Source: CAD feature listing. Evaluate the final solid. Frame: model axes, mm. A direction names the side the tool comes from. Give positions to 0.01 mm unless a question says otherwise; leave off trailing zeros. Loops run counter-clockwise (first coordinate to the right, second up) from the corner with the lowest first, then second, coordinate; pieces in that order, holes last.
```python
from build123d import *

# Parameters (mm, degrees)
SKETCH1_R           = 1.45
SKETCH1_R_2         = 2.6
BOSS_EXTRUDE1_DEPTH = 3
SKETCH1_3_R         = 1.45
BOSS_EXTRUDE2_DEPTH = 29.5
SKETCH1_4_R         = 3
SKETCH1_4_R_2       = 1.45
BOSS_EXTRUDE3_DEPTH = 4
SKETCH5_W           = 14
SKETCH5_H           = 13
SKETCH5_W_2         = 16
SKETCH5_H_2         = 35
CUT_EXTRUDE2_DEPTH  = 3
CUT_EXTRUDE3_REACH  = 150.46


with BuildPart() as part:
    # Sketch1 → Boss-Extrude1 (new body)
    with BuildSketch(Plane.XY):
        with BuildLine():
            Line((-63.5, -59), (63.5, -59))
            ThreePointArc((63.5, -59), (65.621320344, -58.121320344), (66.5, -56))
            Line((66.5, -56), (66.5, 56))
            ThreePointArc((66.5, 56), (65.621320344, 58.121320344), (63.5, 59))
            Line((63.5, 59), (-63.5, 59))
            ThreePointArc((-63.5, 59), (-65.621320344, 58.121320344), (-66.5, 56))
            Line((-66.5, 56), (-66.5, -56))
            ThreePointArc((-66.5, -56), (-65.621320344, -58.121320344), (-63.5, -59))
        make_face()
        with Locations((-59.9, 40.875)):
            Circle(SKETCH1_R, mode=Mode.SUBTRACT)
        with Locations((33.1, 40.875)):
            Circle(SKETCH1_R, mode=Mode.SUBTRACT)
        with Locations((33.1, -30.875)):
            Circle(SKETCH1_R, mode=Mode.SUBTRACT)
        with Locations((-59.9, -30.875)):
            Circle(SKETCH1_R, mode=Mode.SUBTRACT)
        with Locations((-49.9, 11)):
            Circle(SKETCH1_R_2, mode=Mode.SUBTRACT)
        with Locations((51.5, 11)):
            Circle(SKETCH1_R_2, mode=Mode.SUBTRACT)
        with Locations((-49.9, -49)):
            Circle(SKETCH1_R_2, mode=Mode.SUBTRACT)
        with Locations((51.5, -49)):
            Circle(SKETCH1_R_2, mode=Mode.SUBTRACT)
        with BuildLine():
            Line((44.9, 26), (44.9, -16))
            ThreePointArc((44.9, -16), (43.435533906, -19.535533906), (39.9, -21))
            Line((39.9, -21), (9.9, -21))
            ThreePointArc((9.9, -21), (6.364466094, -19.535533906), (4.9, -16))
            Line((4.9, -16), (4.9, 26))
            ThreePointArc((4.9, 26), (6.364466094, 29.535533906), (9.9, 31))
            Line((9.9, 31), (39.9, 31))
            ThreePointArc((39.9, 31), (43.435533906, 29.535533906), (44.9, 26))
        make_face(mode=Mode.SUBTRACT)
        with BuildLine():
            Line((-39.9, 31), (-9.9, 31))
            ThreePointArc((-9.9, 31), (-6.364466094, 29.535533906), (-4.9, 26))
            Line((-4.9, 26), (-4.9, -16))
            ThreePointArc((-4.9, -16), (-6.364466094, -19.535533906), (-9.9, -21))
            Line((-9.9, -21), (-39.9, -21))
            ThreePointArc((-39.9, -21), (-43.435533906, -19.535533906), (-44.9, -16))
            Line((-44.9, -16), (-44.9, 26))
            ThreePointArc((-44.9, 26), (-43.435533906, 29.535533906), (-39.9, 31))
        make_face(mode=Mode.SUBTRACT)
    extrude(amount=-BOSS_EXTRUDE1_DEPTH)

    # Sketch1<3> → Boss-Extrude2 (add)
    with BuildSketch(Plane.XY):
        with BuildLine():
            ThreePointArc((-66.5, 56), (-65.621320344, 58.121320344), (-63.5, 59))
            Line((-63.5, 59), (63.5, 59))
            ThreePointArc((63.5, 59), (65.621320344, 58.121320344), (66.5, 56))
            Line((66.5, 56), (66.5, -56))
            ThreePointArc((66.5, -56), (65.621320344, -58.121320344), (63.5, -59))
            Line((63.5, -59), (-63.5, -59))
            ThreePointArc((-63.5, -59), (-65.621320344, -58.121320344), (-66.5, -56))
            Line((-66.5, -56), (-66.5, 56))
        make_face()
        with Locations(Location((62.5, 55, 0), (0, 0, 180))):
            Circle(SKETCH1_3_R, mode=Mode.SUBTRACT)
        with Locations((-62.5, 55)):
            Circle(SKETCH1_3_R, mode=Mode.SUBTRACT)
        with Locations((62.5, -55)):
            Circle(SKETCH1_3_R, mode=Mode.SUBTRACT)
        with Locations(Location((-62.5, -55, 0), (0, 0, 180))):
            Circle(SKETCH1_3_R, mode=Mode.SUBTRACT)
        with BuildLine():
            ThreePointArc((-62.5, -51.15), (-59.777638892, -52.277638892), (-58.65, -55))
            Line((-58.65, -55), (-58.65, -56))
            Line((-58.65, -56), (58.65, -56))
            Line((58.65, -56), (58.65, -55))
            ThreePointArc((58.65, -55), (59.777638892, -52.277638892), (62.5, -51.15))
            Line((62.5, -51.15), (63.5, -51.15))
            Line((63.5, -51.15), (63.5, 51.15))
            Line((63.5, 51.15), (62.5, 51.15))
            ThreePointArc((62.5, 51.15), (59.777638892, 52.277638892), (58.65, 55))
            Line((58.65, 55), (58.65, 56))
            Line((58.65, 56), (-58.65, 56))
            Line((-58.65, 56), (-58.65, 55))
            ThreePointArc((-58.65, 55), (-59.777638892, 52.277638892), (-62.5, 51.15))
            Line((-62.5, 51.15), (-63.5, 51.15))
            Line((-63.5, 51.15), (-63.5, -51.15))
            Line((-63.5, -51.15), (-62.5, -51.15))
        make_face(mode=Mode.SUBTRACT)
    extrude(amount=BOSS_EXTRUDE2_DEPTH)

    # Sketch1<4> → Boss-Extrude3 (add)
    with BuildSketch(Plane.XY):
        with Locations(Location((-59.9, 40.875, 0), (0, 0, 180))):
            Circle(SKETCH1_4_R)
        with Locations((-59.9, 40.875)):
            Circle(SKETCH1_4_R_2, mode=Mode.SUBTRACT)
        with Locations(Location((33.1, 40.875, 0), (0, 0, 180))):
            Circle(SKETCH1_4_R)
        with Locations((33.1, 40.875)):
            Circle(SKETCH1_4_R_2, mode=Mode.SUBTRACT)
        with Locations(Location((33.1, -30.875, 0), (0, 0, 180))):
            Circle(SKETCH1_4_R)
        with Locations((33.1, -30.875)):
            Circle(SKETCH1_4_R_2, mode=Mode.SUBTRACT)
        with Locations(Location((-59.9, -30.875, 0), (0, 0, 180))):
            Circle(SKETCH1_4_R)
        with Locations((-59.9, -30.875)):
            Circle(SKETCH1_4_R_2, mode=Mode.SUBTRACT)
    extrude(amount=BOSS_EXTRUDE3_DEPTH)

    # Sketch5 → Cut-Extrude2 (cut)
    with BuildSketch(Plane.ZY.offset(66.5)):
        with Locations((11.5, -9.5)):
            Rectangle(SKETCH5_W, SKETCH5_H)
        with BuildLine():
            Line((29.5, -35), (5.5, -35))
            ThreePointArc((5.5, -35), (3.378679656, -35.878679656), (2.5, -38))
            Line((2.5, -38), (2.5, -46))
            ThreePointArc((2.5, -46), (3.378679656, -48.121320344), (5.5, -49))
            Line((5.5, -49), (29.5, -49))
            Line((29.5, -49), (29.5, -35))
        make_face()
        with Locations((21.5, 19.5)):
            Rectangle(SKETCH5_W_2, SKETCH5_H_2)
    extrude(amount=-CUT_EXTRUDE2_DEPTH, mode=Mode.SUBTRACT)

    # Sketch6 → Cut-Extrude3 (cut, up to next)
    with BuildSketch(Plane(origin=(66.5, 0, 0), x_dir=(0, 0, -1), z_dir=(1, 0, 0)), mode=Mode.PRIVATE) as cut_extrude3_sk1:
        with BuildLine():
            Line((-6.5, -45), (-29.5, -45))
            Line((-29.5, -45), (-29.5, -40))
            Line((-29.5, -40), (-6.5, -40))
            ThreePointArc((-6.5, -40), (-5.085786438, -40.585786438), (-4.5, -42))
            Line((-4.5, -42), (-4.5, -43))
            ThreePointArc((-4.5, -43), (-5.085786438, -44.414213562), (-6.5, -45))
        make_face()
    cut_extrude3_tool1 = extrude(cut_extrude3_sk1.sketch, amount=-CUT_EXTRUDE3_REACH, mode=Mode.PRIVATE) & part.part
    add(cut_extrude3_tool1.solids().sort_by_distance((66.5, -42.5, 17.167851))[0], mode=Mode.SUBTRACT)


solid = part.part
```
(1) Reachability of faces 4 (the flat face through (65, -40, 18)), 5 (the flat face through (25, 31, -1)), 6 (the flat face through (25, 57, 29.5)), 7 (the cylindrical face through (-62.76, -31.78, 1.97)) from +Z, -Z, +X, -X, +Y, -Y: full face, straight path, thin tool, end or side. Return the list, or none.
A:
face 4: +Z, +X, -X
face 5: +Z, -Z
face 6: +Z, +X, -X, +Y, -Y
face 7: +Z
(2) Mould query, pull axis Z, two halves, no side actions, for faces 1 (the cylindrical face through (65.64, -58.1, 13.02)), 2 (the flat face through (-65, -10, 18.5)), 3 (the flat face through (62, -55, 0)). Classes: pulls with the +Z half, pulls with the -Z half, needs draft (parallel to the pull), parting line crosses it, or undercut.
A:
face 1: needs draft
face 2: undercut
face 3: pulls with the +Z half
(3) Section D-D, the plane y = 11. Return the cut outline in (x, z), then the cut area to 3 significant figures.
A:
outline: (-66.5, -3) - (-52.5, -3) - (-52.5, 0) - (-63.5, 0) - (-63.5, 13.5) - (-66.5, 13.5) - close; (-47.3, -3) - (-44.9, -3) - (-44.9, 0) - (-47.3, 0) - close; (-4.9, -3) - (4.9, -3) - (4.9, 0) - (-4.9, 0) - close; (44.9, -3) - (48.9, -3) - (48.9, 0) - (44.9, 0) - close; (54.1, -3) - (66.5, -3) - (66.5, 29.5) - (63.5, 29.5) - (63.5, 0) - (54.1, 0) - close
area: 257 mm2
(4) Section B-B, the plane x = -49.9. Return the cut outline in (y, z).
A:
outline: (-59, -3) - (-51.6, -3) - (-51.6, 0) - (-56, 0) - (-56, 29.5) - (-59, 29.5) - close; (-46.4, -3) - (8.4, -3) - (8.4, 0) - (-46.4, 0) - close; (13.6, -3) - (59, -3) - (59, 29.5) - (56, 29.5) - (56, 0) - (13.6, 0) - close
(5) First-contact query: pin 1 (3.5 mm diameter, centred on x = -65.5, z = 22, fed in from +Y); pin 2 (10 mm diameter, centred on x = 50, y = 45, fed in from +Z); pin 3 (4.5 mm diameter, centred on x = 33.1, y = 40.875, fed in from +Z). Flat tips, straight axial feed; report the tip coordinate or a pass-through.
A:
pin 1: stops at y = 58.99
pin 2: stops at z = 0
pin 3: stops at z = 4
(6) Section C-C, the plane z = 15.5. Count the separate pieces of the cut face and the enclosed holes in it, then the cut area to 3 significant figures.
A:
separate pieces: 4
enclosed holes: 4
area: 1,320 mm2
(7) Section A-A, the plane y = -7.5. Return the cut outline in (x, z).
A:
outline: (-66.5, -3) - (-44.9, -3) - (-44.9, 0) - (-63.5, 0) - (-63.5, 4.5) - (-66.5, 4.5) - close; (-66.5, 18.5) - (-63.5, 18.5) - (-63.5, 29.5) - (-66.5, 29.5) - close; (-4.9, -3) - (4.9, -3) - (4.9, 0) - (-4.9, 0) - close; (44.9, -3) - (66.5, -3) - (66.5, 29.5) - (63.5, 29.5) - (63.5, 0) - (44.9, 0) - close
(8) Ray query, line 1 along Y through (x, z) = (51.5, -1.9); line 2 along X through (y, z) = (-48, 1); line 3 along Y through (x, z) = (33.1, 2.95) (3 decimals). Return the intervals inside material, ascending.
A:
line 1: y = -59 to -51.6, -46.4 to 8.4, 13.6 to 59
line 2: x = -66.5 to -63.5, 63.5 to 66.5
line 3: y = -59 to -56, -33.875 to -32.325, -29.425 to -27.875, 37.875 to 39.425, 42.325 to 43.875, 56 to 59
